Model file for the job. Use its own axes, mm. A direction names the side the tool comes from. Round coordinates to 2 decimals unless told otherwise and drop trailing zeros. Loops run counter-clockwise (first coordinate to the right, second up) from the corner with the lowest first, then second, coordinate; pieces in that order, holes last. Notation, with made-up numbers: (34.5, 80) -> (75.5, 80) arc R16 ccw to (75.5, 111) -> close; hole circle Ø9 at (9, 63). An arc over 180 degrees is marked (long way). Use a Markdown table: item, result.
from build123d import *

# Parameters (mm, degrees)
SKETCH_1_R           = 25
EXTRUDE_1_DEPTH      = 5
SKETCH_2_R           = 7.5
EXTRUDE_2_DEPTH      = 9
SKETCH_3_R           = 3
EXTRUDE_3_DEPTH      = 5
FILLET_1_R           = 1
EXTRUDE_4_DEPTH      = 1
EXTRUDE_4_DEPTH_BACK = 1
FILLET_2_R           = 0.25
EXTRUDE_5_DEPTH      = 5
CUT_EXTRUDE_1_DEPTH  = 1
SKETCH_7_R           = 1
CUT_EXTRUDE_2_DEPTH  = 21


with BuildPart() as part:
    # Эскиз1 → Бобышка-Вытянуть1 (new body)
    with BuildSketch(Plane.XY):
        Circle(SKETCH_1_R)
    extrude(amount=EXTRUDE_1_DEPTH)

    # Эскиз2 → Бобышка-Вытянуть2 (add)
    with BuildSketch(Plane.XY.offset(5)):
        Circle(SKETCH_2_R)
    extrude(amount=EXTRUDE_2_DEPTH)

    # Эскиз3 → Бобышка-Вытянуть3 (add)
    with BuildSketch(Plane.XY.offset(5)):
        with Locations((15.5, 0)):
            Circle(SKETCH_3_R)
        with Locations((-15.5, 0)):
            Circle(SKETCH_3_R)
    extrude(amount=EXTRUDE_3_DEPTH)

    # Скругление1
    fillet_1_edges = [part.edges().sort_by_distance(p)[0] for p in [
        (-7.5, 0, 14),
    ]]
    fillet(fillet_1_edges, radius=FILLET_1_R)

    # Эскиз4 → Бобышка-Вытянуть4 (add, two sides: drawn at the far end of the back side and taken through both)
    with BuildSketch(Plane(origin=(0, 0, 0), x_dir=(1, 0, 0), z_dir=(0, 1, 0)).offset(-EXTRUDE_4_DEPTH_BACK)):
        Polygon((-15.889303471, -8.350739368), (-5.011906667, -12.039097177), (-5.011906667, -5), (-15.889303471, -5), align=None)
        Polygon((5.011906667, -12.039097177), (5.011906667, -5), (15.889303471, -5), (15.889303471, -8.350739368), align=None)
    extrude(amount=EXTRUDE_4_DEPTH + EXTRUDE_4_DEPTH_BACK)

    # Скругление2
    fillet_2_edges = [part.edges().sort_by_distance(p)[0] for p in [
        (-18.5, 0, 10),
        (12.5, 0, 10),
    ]]
    fillet(fillet_2_edges, radius=FILLET_2_R)

    # Эскиз5 → Бобышка-Вытянуть5 (add)
    with BuildSketch(Plane.XY.offset(5)):
        with BuildLine():
            Line((17.67766953, 18.384776311), (17.015216986, 17.722323767))
            Line((17.015216986, 17.722323767), (17.709176341, 17.028364412))
            Line((17.709176341, 17.028364412), (18.377652971, 17.670686903))
            ThreePointArc((18.377652971, 17.670686903), (18.388285388, 18.381232054), (17.67766953, 18.384776311))
        make_face()
    extrude(amount=-EXTRUDE_5_DEPTH)

    # Эскиз6 → Вырез-Вытянуть1 (cut)
    with BuildSketch(Plane.XY.offset(5)):
        with BuildLine():
            Line((-5.5, 9.5), (5.5, 9.5))
            ThreePointArc((5.5, 9.5), (6.914213562, 10.085786438), (7.5, 11.5))
            Line((7.5, 11.5), (7.5, 17.5))
            ThreePointArc((7.5, 17.5), (6.914213562, 18.914213562), (5.5, 19.5))
            Line((5.5, 19.5), (-5.5, 19.5))
            ThreePointArc((-5.5, 19.5), (-6.914213562, 18.914213562), (-7.5, 17.5))
            Line((-7.5, 17.5), (-7.5, 11.5))
            ThreePointArc((-7.5, 11.5), (-6.914213562, 10.085786438), (-5.5, 9.5))
        make_face()
    extrude(amount=-CUT_EXTRUDE_1_DEPTH, mode=Mode.SUBTRACT)

    # Эскиз7 → Вырез-Вытянуть2 (cut)
    with BuildSketch(Plane.XY.offset(4)):
        with Locations((-2.5, 14.5)):
            Circle(SKETCH_7_R)
        with Locations((2.5, 14.5)):
            Circle(SKETCH_7_R)
    extrude(amount=-CUT_EXTRUDE_2_DEPTH, mode=Mode.SUBTRACT)


solid = part.part
Q1. Drill centre lines: L1, parallel to X at y = -2, z = 8; L2, parallel to Z at x = -7.5, y = -17; L3, parallel to Y at x = 2.5, z = 1.8. Where is each one in solid material? Low to high. Write a range as from..to.
Results list:
| item | result |
|---|---|
| L1 | x = -17.74..-13.26, -7.23..7.23, 13.26..17.74 |
| L2 | z = 0..5 |
| L3 | y = -24.87..13.5, 15.5..24.87 |
Q2. Band-saw the part on A-A, the plane x = 0. Give the cut face in (y, z), plus the area to 3 significant figures.
Results list:
| item | result |
|---|---|
| outline | (-25, 0) -> (25, 0) -> (25, 5) -> (19.5, 5) -> (19.5, 4) -> (9.5, 4) -> (9.5, 5) -> (7.5, 5) -> (7.5, 13) arc R1 ccw to (6.5, 14) -> (-6.5, 14) arc R1 ccw to (-7.5, 13) -> (-7.5, 5) -> (-25, 5) -> close |
| area | 375 mm² |
Q3. Band-saw the part on B-B, the plane y = 14.5. Give the cut face in (x, z), plus the area to 3 significant figures.
Results list:
| item | result |
|---|---|
| outline | (-20.37, 0) -> (-3.5, 0) -> (-3.5, 4) -> (-7.5, 4) -> (-7.5, 5) -> (-20.37, 5) -> close; (-1.5, 0) -> (1.5, 0) -> (1.5, 4) -> (-1.5, 4) -> close; (3.5, 0) -> (20.37, 0) -> (20.37, 5) -> (7.5, 5) -> (7.5, 4) -> (3.5, 4) -> close |
| area | 173 mm² |
Q4. Flat gauge pins, fed straight in: pin 1 (0.5 mm diameter, centred on y = 13.5, z = 4.5, fed in from +X); pin 2 (1.6 mm diameter, centred on x = -10.5, z = 8, fed in from +Y); pin 3 (1.6 mm diameter, centred on x = -10, z = 8.5, fed in from -Y); pin 4 (1.6 mm diameter, centred on x = 2.5, y = 14.5, fed in from -Z). Where does each tip first touch, or does it go through?
Results list:
| item | result |
|---|---|
| pin 1 | stops at x = 21.2 |
| pin 2 | stops at y = 1 |
| pin 3 | stops at y = -1 |
| pin 4 | passes through |
Q5. Band-saw the part on D-D, the plane z = 1. Give the cut face in (x, y), plus the area to 3 significant figures.
Results list:
| item | result |
|---|---|
| outline | (17.32, 18.03) arc R25 ccw (long way) to (18.02, 17.33) -> (18.38, 17.67) arc R0.5 ccw (long way) to (17.68, 18.38) -> close; hole circle Ø2 at (-2.5, 14.5); hole circle Ø2 at (2.5, 14.5) |
| area | 1,960 mm² |
Q6. Band-saw the part on C-C, the plane z = 8.5. Give the cut face in (x, y), plus the area to 3 significant figures.
Results list:
| item | result |
|---|---|
| outline | (-12.67, -1) -> (-7.43, -1) arc R7.5 ccw to (7.43, -1) -> (12.67, -1) arc R3 ccw (long way) to (12.67, 1) -> (7.43, 1) arc R7.5 ccw to (-7.43, 1) -> (-12.67, 1) arc R3 ccw (long way) to start |
| area | 254 mm² |
Q7. Tool access for faces 1 (the face through (-6.9, 18.93, 4.51)), 2 (the face through (-16, 0, 10)), 3 (the face through (-10, -1, 7)): list every direction of +Z, -Z, +X, -X, +Y, -Y with a clear straight run to the whole face (end or side of a thin tool).
Results list:
| item | result |
|---|---|
| face 1 | +Z |
| face 2 | +Z, -X, +Y, -Y |
| face 3 | +Z, -Y |
